Geometry: final body of the model. Coordinates: model frame, mm. Give positions to 0.01 mm unless a question says otherwise; leave off trailing zeros. Loops run counter-clockwise (first coordinate to the right, second up) from the corner with the lowest first, then second, coordinate; pieces in that order, holes last. Notation, with made-up numbers: (-32.5, 65.5) -> (26.5, 65.5) arc R18 cw to (26.5, 84.5) -> close; hole circle Ø10 at (59.5, -35). An arc over 180 degrees is marked (long way). Answer in a Markdown table with one row per item. Add a question column.
from build123d import *

# Parameters (mm, degrees)
F0_W     = 226.934584
F0_H     = 132.857451
F0_R     = 3
F0_R_2   = 15.497899
F0_R_3   = 12.7
F1_DEPTH = 5.08
F2_R     = 23.8125


with BuildPart() as f1:
    # F0 (on Top) → F1 (new body)
    with BuildSketch(Plane.XY):
        with Locations((-45.531327, 1.507239)):
            Rectangle(F0_W, F0_H)
        with Locations((0, -32.000012)):
            Circle(F0_R, mode=Mode.SUBTRACT)
        Circle(F0_R_2, mode=Mode.SUBTRACT)
        with Locations((-27.712823, 16.000006)):
            Circle(F0_R, mode=Mode.SUBTRACT)
        with Locations((27.712823, 16.000006)):
            Circle(F0_R, mode=Mode.SUBTRACT)
        with Locations((44.123465, 44.123465)):
            Circle(F0_R_3, mode=Mode.SUBTRACT)
    extrude(amount=F1_DEPTH)

    # F2
    f2_edges = [f1.edges().sort_by_distance(p)[0] for p in [
        (67.935965, 67.935965, 2.54),
    ]]
    fillet(f2_edges, radius=F2_R)


solid = f1.part
(1) Cut plane A-A on y = 0. Return the cut outline in (x, z), then the cut area to 3 significant figures.
(2) Material intervals for line 1 along Y through (x, z) = (0, 2.5); line 2 along Y through (x, z) = (27.5, 1.75); line 3 along X through (y, z) = (55, 4.65), sorted ascending. Write a range as from..to.
(3) Cut plane D-D on z = 2.8. Return the cut outline in (x, y) (1 decimal), then the cut area to 3 significant figures.
(4) Pin query (flat end, axial travel): pin 1 Ø9.5 at (x, y) = (0, -32) entering from +Z. Return the tip coordinate at first contact, or that it passes through.
(5) Cut plane C-C on x = 27.5. Return the cut outline in (y, z).
(6) Draft query along Y for faces 1 (the flat face through (-158.999, 1, 3)), 2 (the flat face through (-59, 67.936, 3)), 3 (the cylindrical face through (-30.09, 14.17, 2.5)). Return one class per face: +Y half, -Y half, draft (parallel to the pull), parting line (faces both ways), or undercut.
(7) Cut plane B-B on x = 0. Return the cut outline in (y, z), then the cut area to 3 significant figures.
Answer list:
| question | item | result |
|---|---|---|
| 1 | outline | (-159, 0) -> (-15.5, 0) -> (-15.5, 5.08) -> (-159, 5.08) -> close; (15.5, 0) -> (67.94, 0) -> (67.94, 5.08) -> (15.5, 5.08) -> close |
| 1 | area | 995 mm² |
| 2 | line 1 | y = -64.92..-35, -29..-15.5, 15.5..67.94 |
| 2 | line 2 | y = -64.92..13.01, 18.99..67.94 |
| 2 | line 3 | x = -159..37.57, 50.68..65.31 |
| 3 | outline | (-159, -64.9) -> (67.9, -64.9) -> (67.9, 44.1) arc R23.8 ccw to (44.1, 67.9) -> (-159, 67.9) -> close; hole circle Ø6 at (-27.7, 16); hole circle Ø31 at (0, 0); hole circle Ø6 at (0, -32); hole circle Ø6 at (27.7, 16); hole circle Ø25.4 at (44.1, 44.1) |
| 3 | area | 28,700 mm² |
| 4 | pin 1 | stops at z = 5.08 |
| 5 | outline | (-64.92, 0) -> (13.01, 0) -> (13.01, 5.08) -> (-64.92, 5.08) -> close; (18.99, 0) -> (67.94, 0) -> (67.94, 5.08) -> (18.99, 5.08) -> close |
| 6 | face 1 | draft |
| 6 | face 2 | +Y half |
| 6 | face 3 | undercut |
| 7 | outline | (-64.92, 0) -> (-35, 0) -> (-35, 5.08) -> (-64.92, 5.08) -> close; (-29, 0) -> (-15.5, 0) -> (-15.5, 5.08) -> (-29, 5.08) -> close; (15.5, 0) -> (67.94, 0) -> (67.94, 5.08) -> (15.5, 5.08) -> close |
| 7 | area | 487 mm² |
